Part model, mm, in its own coordinate system. A direction names the side the tool comes from. Give positions to 0.01 mm unless a question says otherwise; leave off trailing zeros. Order: outer loops, then holes, each group sorted by start corner. A loop starts at its lowest first (then second) coordinate and runs counter-clockwise, first axis right, second up. Notation, with made-up numbers: M 84.5,-36.75 L 103.5,-36.75 A23 cw 103.5,-24.75 Z; hole C -8.75,-6.75 d6. An arc over 180 degrees is marked long. Return JSON: item names as keys, results as strings.
from build123d import *

# Parameters (mm, degrees)
BOSS_EXTRU_1_DEPTH   = 5
D_GAGEMENT_M41_D     = 4.3
D_GAGEMENT_M41_DEPTH = 10
D_GAGEMENT_M41_TIP   = 1.291850331


with BuildPart() as part:
    # Esquisse1 → Boss.-Extru.1 (new body)
    with BuildSketch(Plane.XY):
        with BuildLine():
            Line((-37.5, -41.5), (37.5, -41.5))
            ThreePointArc((37.5, -41.5), (40.328427125, -40.328427125), (41.5, -37.5))
            Line((41.5, -37.5), (41.5, 37.5))
            ThreePointArc((41.5, 37.5), (40.328427125, 40.328427125), (37.5, 41.5))
            Line((37.5, 41.5), (-37.5, 41.5))
            ThreePointArc((-37.5, 41.5), (-40.328427125, 40.328427125), (-41.5, 37.5))
            Line((-41.5, 37.5), (-41.5, -37.5))
            ThreePointArc((-41.5, -37.5), (-40.328427125, -40.328427125), (-37.5, -41.5))
        make_face()
        with BuildLine():
            Line((-14.5, -33.5), (14.5, -33.5))
            ThreePointArc((14.5, -33.5), (17.328427125, -32.328427125), (18.5, -29.5))
            Line((18.5, -29.5), (18.5, -29))
            ThreePointArc((18.5, -29), (20.257359313, -24.757359313), (24.5, -23))
            Line((24.5, -23), (29.5, -23))
            ThreePointArc((29.5, -23), (32.328427125, -21.828427125), (33.5, -19))
            Line((33.5, -19), (33.5, 19))
            ThreePointArc((33.5, 19), (32.328427125, 21.828427125), (29.5, 23))
            Line((29.5, 23), (24.5, 23))
            ThreePointArc((24.5, 23), (20.257359313, 24.757359313), (18.5, 29))
            Line((18.5, 29), (18.5, 29.5))
            ThreePointArc((18.5, 29.5), (17.328427125, 32.328427125), (14.5, 33.5))
            Line((14.5, 33.5), (-14.5, 33.5))
            ThreePointArc((-14.5, 33.5), (-17.328427125, 32.328427125), (-18.5, 29.5))
            Line((-18.5, 29.5), (-18.5, 29))
            ThreePointArc((-18.5, 29), (-20.257359313, 24.757359313), (-24.5, 23))
            Line((-24.5, 23), (-29.5, 23))
            ThreePointArc((-29.5, 23), (-32.328427125, 21.828427125), (-33.5, 19))
            Line((-33.5, 19), (-33.5, -19))
            ThreePointArc((-33.5, -19), (-32.328427125, -21.828427125), (-29.5, -23))
            Line((-29.5, -23), (-24.5, -23))
            ThreePointArc((-24.5, -23), (-20.257359313, -24.757359313), (-18.5, -29))
            Line((-18.5, -29), (-18.5, -29.5))
            ThreePointArc((-18.5, -29.5), (-17.328427125, -32.328427125), (-14.5, -33.5))
        make_face(mode=Mode.SUBTRACT)
    extrude(amount=BOSS_EXTRU_1_DEPTH)

    # Dégagement M41
    with Locations(Plane.XY.offset(5)):
        with Locations((-37.5, 37.5), (37.5, 37.5), (37.5, -37.5), (-37.5, -37.5), (-24.5, 29), (24.5, 29), (24.5, -29), (-24.5, -29)):
            Hole(D_GAGEMENT_M41_D / 2, depth=D_GAGEMENT_M41_DEPTH)
            with Locations((0, 0, -(D_GAGEMENT_M41_DEPTH + D_GAGEMENT_M41_TIP / 2))):  # 118° drill point
                Cone(0, D_GAGEMENT_M41_D / 2, D_GAGEMENT_M41_TIP, mode=Mode.SUBTRACT)


solid = part.part
Q1. Probe line 1 along Y through (x, z) = (24.5, 2.05); line 2 along Y through (x, z) = (37.5, 1.8); line 3 along X through (y, z) = (-16.5, 4.1). List the from-to ranges inside material, lowest first.
Established:
{"line 1": "y = -41.5 to -31.15, -26.85 to -23, 23 to 26.85, 31.15 to 41.5", "line 2": "y = -41.5 to -39.65, -35.35 to 35.35, 39.65 to 41.5", "line 3": "x = -41.5 to -33.5, 33.5 to 41.5"}
Q2. 3-axis set-ups, long thin cutter, end or side, ignore diameter. For faces 1 (the flat face through (-19, 28, 0)), 2 (the cylindrical face through (-20.304, -24.711, 2.465)): which of +Z, -Z, +X, -X, +Y, -Y reach the whole face in a straight line?
Established:
{"face 1": "-Z, +X, -X, +Y, -Y", "face 2": "+Z, -Z"}
Q3. Band-saw the part on C-C (z = 3.6). Give the number of separate pieces and of enclosed holes in the cut face, then the cut area to 3 significant figures.
Established:
{"separate pieces": "1", "enclosed holes": "9", "area": "2,900 mm²"}
Q4. Pin check, flat tips, straight feed: pin 1 (4 mm diameter, centred on x = -37.5, y = 37.5, fed in from -Z); pin 2 (12 mm diameter, centred on x = -28, y = -0.5, fed in from -Z). Stop position of each tip, or through.
Established:
{"pin 1": "passes through", "pin 2": "stops at z = 0"}
Q5. Band-saw the part on A-A (x = -1). Give the cut face in (y, z), then the cut area to 3 significant figures.
Established:
{"outline": "M -41.5,0 L -33.5,0 L -33.5,5 L -41.5,5 Z; M 33.5,0 L 41.5,0 L 41.5,5 L 33.5,5 Z", "area": "80.0 mm²"}
Q6. Two-plate mould, pull along Y, no slides. Class faces 3 (the cylindrical face through (36.34, 39.31, 2.46)), 4 (the cylindrical face through (40.359, 40.297, 2.465)), 5 (the cylindrical face through (-40.359, -40.297, 2.465)): +Y half, -Y half, draft (parallel to the pull), parting line (faces both ways), or undercut.
Established:
{"face 3": "undercut", "face 4": "+Y half", "face 5": "-Y half"}
